Could you check a few things on this model? Use its own coordinates, in mm. Face numbers are marked on the shaded views. A direction names the side the tool comes from. Give positions to 0.01 mm unless a question says otherwise; leave off trailing zeros. Order: outer loops, then holes, each group sorted by start corner. A loop starts at its lowest first (then second) coordinate and runs counter-clockwise, first axis right, second up. Notation, with made-up numbers: M -23.5,18.5 L 14.5,18.5 A19 ccw 14.5,53.5 Z; hole C 66.25,86 d10. An arc over 180 degrees is marked long. Return JSON: item names as keys, results as strings. Group by question number.
```python
from build123d import *

# Parameters (mm, degrees)
F1_DEPTH = 28
F2_R     = 1.5
F3_DEPTH = 3
F4_R     = 1.5
F5_DEPTH = 5


with BuildPart() as f1:
    # F0 (on Front) → F1 (new body)
    with BuildSketch(Plane.XZ):
        Polygon((0.116138, -3.635452), (3.206463, -1.717148), (3.090325, 1.918304), (-0.116138, 3.635452), (-3.206463, 1.717148), (-3.090325, -1.918304), align=None)
    extrude(amount=-F1_DEPTH)

    # F2 (on face) → F3 (join)
    with BuildSketch(Plane.XZ):
        Circle(F2_R)
    extrude(amount=F3_DEPTH)

    # F4 (on face) → F5 (join)
    with BuildSketch(Plane(origin=(0, 28, 0), x_dir=(-1, 0, 0), z_dir=(0, 1, 0))):
        Circle(F4_R)
    extrude(amount=F5_DEPTH)


solid = f1.part
```
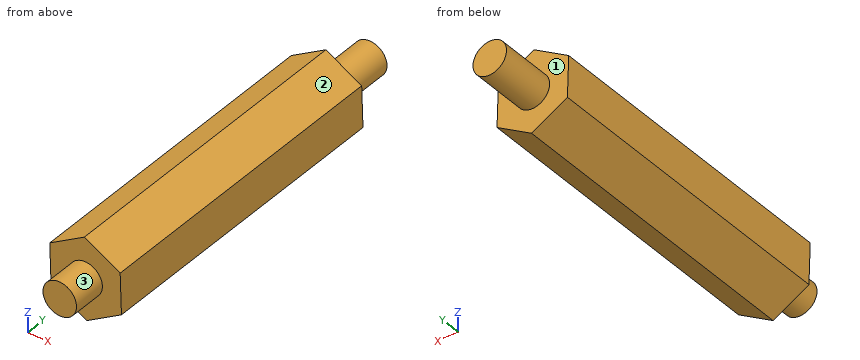
1. Imagine slicing it at D-D, the plane x = 2.75. Please give me the cut outline in (y, z).
2. I need wall thicknesses on L1, parallel to Y at x = -0.5, z = -3; L2, parallel to X at y = 11, z = 1.25; L3, parallel to Z at x = 1.25, y = 8. Which ranges of each line are inside material? Lowest first, please. Write a range as from..to.
3. Which directions (+Z, -Z, +X, -X, +Y, -Y) give clear straight access to the entire face, cutting with the end or side of a thin tool? Please do the marked faces 1, 2 and 3.
4. For pin 1 (3 mm diameter, centred on y = 9, z = -0.5, fed in from -X); pin 2 (1 mm diameter, centred on x = 0.5, y = 27, fed in from +Z); pin 3 (1 mm diameter, centred on y = 17.5, z = -1, fed in from +X), each with a flat end and sliding along its axis, tell me the tip position at first contact or that it passes through.
5. Imagine slicing it at A-A, the plane y = 14. Please give me the cut outline in (x, z).
6. Imagine slicing it at C-C, the plane x = 1. Please give me the cut outline in (y, z).
7. Imagine slicing it at B-B, the plane z = 0. Please give me the cut outline in (x, y), plus the area to 3 significant figures.
Values:
{
 "1": {"outline": "M 0,-2 L 28,-2 L 28,2.1 L 0,2.1 Z"},
 "2": {"L1": "y = 0..28", "L2": "x = -3.19..3.11", "L3": "z = -2.93..2.9"},
 "3": {"face 1": "+Y", "face 2": "+Z, +X, +Y, -Y", "face 3": "-Y"},
 "4": {"pin 1": "stops at x = -3.18", "pin 2": "stops at z = 3.57", "pin 3": "stops at x = 3.2"},
 "5": {"outline": "M -3.21,1.72 L -3.09,-1.92 L 0.12,-3.64 L 3.21,-1.72 L 3.09,1.92 L -0.12,3.64 Z"},
 "6": {"outline": "M -3,-1.12 L 0,-1.12 L 0,-3.09 L 28,-3.09 L 28,-1.12 L 33,-1.12 L 33,1.12 L 28,1.12 L 28,3.04 L 0,3.04 L 0,1.12 L -3,1.12 Z"},
 "7": {"outline": "M -3.15,0 L -1.5,0 L -1.5,-3 L 1.5,-3 L 1.5,0 L 3.15,0 L 3.15,28 L 1.5,28 L 1.5,33 L -1.5,33 L -1.5,28 L -3.15,28 Z", "area": "200 mm²"}
}
